The listing builds one solid part. Answer for the finished solid, in the listing's coordinates (mm). A direction names the side the tool comes from. Coordinates: 2 decimals unless noted, no trailing zeros. Order: outer loops, then holes, each group sorted by start corner. A loop starts at its lowest first (then second) coordinate and runs counter-clockwise, first axis right, second up. Notation, with made-up numbers: (70.25, -38) -> (103.25, -38) arc R24 cw to (103.25, -12) -> close; hole circle Ø2 at (10.25, 48.5). An arc over 180 degrees is marked (long way). Return JSON: item names as keys, results as strings.
Autodesk Inventor part; units mm, degrees
ref_plane "Work Plane1" through (-100.0106, -952.6394, 1035.6952) normal (0, 1, 0) x (-1, 0, 0)
ref_plane "YZ Plane" through (0, 0, 0) normal (1, 0, 0) x (0, 1, 0)
ref_plane "XZ Plane" through (0, 0, 0) normal (0, 1, 0) x (-1, 0, 0)
ref_plane "Work Plane1" through (-100.0106, -952.6394, 1035.6952) normal (0, 1, 0) x (-1, 0, 0)
sketch "Sketch3" plane through (-100.0106, -952.6394, 1035.6952) normal (0, 1, 0) x (-1, 0, 0)
  circle A0 centre (0, 0) radius 4.7625
  circle A1 centre (0, 0) radius 4.0005
sketch3d "3D Sketch1"
  line L0 (-100.0106, -952.6394, 1035.6952) -> (-100.0106, -915.4309, 1035.6952)
  arc A0 (-100.0106, -915.4309, 1035.6952) -> (-94.0107, -909.431, 1035.6952) centre (-94.0107, -915.4309, 1035.6952) ccw
  line L1 (-94.0107, -909.431, 1035.6952) -> (137.3561, -909.431, 1035.6952)
  dimension "d4" = 5.9999
sweep "Sweep1" add profiles "Sketch3" path "3D Sketch1"
equation "\"OD\" = 9.525"
equation "\"t\" = 0.762"
equation "\"L\" = PL"
equation "\"ID\" = 8.001"
equation "\"PL\" = 278.003"
equation "\"Size_Designation\" = 1.2345"
properties material "Copper"
1. The part is cut by section C-C on x = 9. Give the vertices of the cut face in (y, z) (1 decimal).
Answer block:
{"outline": "circle Ø9.5 at (-909.4, 1035.7); hole circle Ø8 at (-909.4, 1035.7)"}
2. For faces 1 (the face through (137.356, -913, 1033)), 2 (the face through (-98.978, -933.775, 1031.046)), determine the directions among +Z, -Z, +X, -X, +Y, -Y from which every point of the face is accessible in a straight line to the end or side of a thin tool.
Answer block:
{"face 1": "+Z, -Z, +X, +Y, -Y", "face 2": "-Y"}
3. Each of these flat-tipped pins is pushed along its axis until it touches: pin 1 Ø3 at (y, z) = (-941, 1037.5) entering from +X; pin 2 Ø12 at (x, y) = (8, -916) entering from -Z; pin 3 Ø3 at (y, z) = (-923, 1039) entering from -X. Where does it stop, or does it pass through?
Answer block:
{"pin 1": "stops at x = -95.26", "pin 2": "stops at z = 1030.97", "pin 3": "stops at x = -104.42"}
4. Determine the mould class of faces 3 (the face through (-98, -952.639, 1032)), 4 (the face through (-97.062, -933.775, 1038.399)), 5 (the face through (23.29, -912.38, 1038.4)), 6 (the face through (23.29, -913.21, 1032.8)) for opening direction Y: pulls with the +Y half, pulls with the -Y half, needs draft (parallel to the pull), parting line crosses it, or undercut.
Answer block:
{"face 3": "pulls with the -Y half", "face 4": "needs draft", "face 5": "undercut", "face 6": "parting line crosses it"}
5. The part is cut by section B-B on y = -932.5. Give the vertices of the cut face in (x, z) (1 decimal), and give its area (3 significant figures).
Answer block:
{"outline": "circle Ø9.5 at (-100, 1035.7); hole circle Ø8 at (-100, 1035.7)", "area": "21.0 mm2"}
6. Consider line 1 (X direction, y = -934.5, z = 1036.25); line 2 (X direction, y = -916, z = 1035.75); line 3 (Z direction, x = 126, y = -909). Determine where each line is inside the solid, lowest interval first. Write a range as from..to.
Answer block:
{"line 1": "x = -104.74..-103.97, -96.05..-95.28", "line 2": "x = -104.77..-104.01, -96.01..-95.25", "line 3": "z = 1030.95..1031.72, 1039.67..1040.44"}
7. The part is cut by section A-A on z = 1038. Give the vertices of the cut face in (x, y), and give its area (3 significant figures).
Answer block:
{"outline": "(-104.18, -952.64) -> (-103.28, -952.64) -> (-103.28, -915.43) arc R9.27 cw to (-94.01, -906.16) -> (137.36, -906.16) -> (137.36, -905.26) -> (-94.01, -905.26) arc R10.17 ccw to (-104.18, -915.43) -> close; (-96.74, -952.64) -> (-95.84, -952.64) -> (-95.84, -915.43) arc R1.83 cw to (-94.01, -913.6) -> (137.36, -913.6) -> (137.36, -912.7) -> (-94.01, -912.7) arc R2.73 ccw to (-96.74, -915.43) -> close", "area": "499 mm2"}
